Verification items for the finished model (mm, model axes). Face numbers are marked on the shaded views. A direction names the side the tool comes from. Give positions to 0.01 mm unless a question says otherwise; leave off trailing zeros. Loops run counter-clockwise (first coordinate to the right, second up) from the corner with the lowest first, then second, coordinate; pieces in that order, holes last. Notation, with made-up numbers: M 60.25,-32.5 L 79.25,-32.5 A24 ccw 79.25,-12.5 Z; hole C 13.5,12.25 d1. An arc over 180 degrees is marked long. Use a Markdown table: item, result.
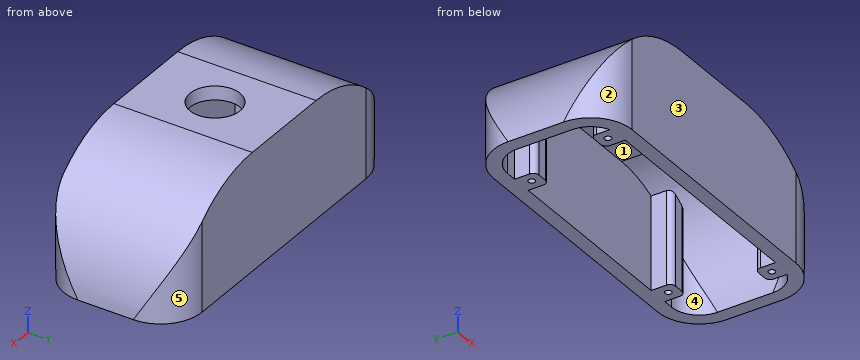
from build123d import *

# Parameters (mm, degrees)
BOSS_EXTRUDE2_DEPTH      = 44.45
BOSS_EXTRUDE2_DEPTH_BACK = 19.05
CUT_EXTRUDE_THIN1_DEPTH  = 104.419258966
SHELL1_T                 = -6.35
SKETCH5_R                = 11.5
CUT_EXTRUDE1_DEPTH       = 6.35
BOSS_EXTRUDE3_REACH      = 105.419
SKETCH8_W                = 9.525
SKETCH8_H                = 9.525
SKETCH8_R                = 1.5
FILLET1_R                = 2.54


with BuildPart() as part:
    # Sketch3 → Boss-Extrude2 (new, two sides: drawn at the far end of the back side and taken through both)
    with BuildSketch(Plane(origin=(0, 0, 0), x_dir=(1, 0, 0), z_dir=(0, 1, 0)).offset(-BOSS_EXTRUDE2_DEPTH_BACK)):
        with BuildLine():
            Line((-76.2, 0), (76.2, 0))
            ThreePointArc((76.2, 0), (60.391088515, -38.166088515), (22.225, -53.975))
            Line((22.225, -53.975), (-22.225, -53.975))
            ThreePointArc((-22.225, -53.975), (-60.391088515, -38.166088515), (-76.2, 0))
        make_face()
    extrude(amount=BOSS_EXTRUDE2_DEPTH + BOSS_EXTRUDE2_DEPTH_BACK)

    # Sketch4 → Cut-Extrude-Thin1 (cut, through all)
    with BuildSketch(Plane.XY.offset(53.975)):
        with BuildLine():
            Line((88.9, 25.4), (88.9, 0))
            ThreePointArc((88.9, 0), (79.600640303, -22.450640303), (57.15, -31.75))
            Line((57.15, -31.75), (-57.15, -31.75))
            ThreePointArc((-57.15, -31.75), (-79.600640303, -22.450640303), (-88.9, 0))
            Line((-88.9, 0), (-88.9, 25.4))
            ThreePointArc((-88.9, 25.4), (-79.600640303, 47.850640303), (-57.15, 57.15))
            Line((-57.15, 57.15), (57.15, 57.15))
            ThreePointArc((57.15, 57.15), (79.600640303, 47.850640303), (88.9, 25.4))
        make_face()
        with BuildLine():
            Line((76.2, 25.4), (76.2, 0))
            ThreePointArc((76.2, 0), (70.620384182, -13.470384182), (57.15, -19.05))
            Line((57.15, -19.05), (-57.15, -19.05))
            ThreePointArc((-57.15, -19.05), (-70.620384182, -13.470384182), (-76.2, 0))
            Line((-76.2, 0), (-76.2, 25.4))
            ThreePointArc((-76.2, 25.4), (-70.620384182, 38.870384182), (-57.15, 44.45))
            Line((-57.15, 44.45), (57.15, 44.45))
            ThreePointArc((57.15, 44.45), (70.620384182, 38.870384182), (76.2, 25.4))
        make_face(mode=Mode.SUBTRACT)
    extrude(amount=-CUT_EXTRUDE_THIN1_DEPTH, mode=Mode.SUBTRACT)

    # Shell1
    shell1_openings = [part.faces().sort_by_distance(p)[0] for p in [
        (0, 12.7, 0),
    ]]
    offset(amount=SHELL1_T, openings=shell1_openings)

    # Sketch5 → Cut-Extrude1 (cut)
    with BuildSketch(Plane.XY.offset(53.975)):
        with Locations((0, 12.7)):
            Circle(SKETCH5_R)
    extrude(amount=-CUT_EXTRUDE1_DEPTH, mode=Mode.SUBTRACT)

    # Sketch8 → Boss-Extrude3 (add, up to next)
    with BuildSketch(Plane(origin=(0, 0, 0), x_dir=(-1, 0, 0), z_dir=(0, 0, -1)), mode=Mode.PRIVATE) as boss_extrude3_sk1:
        with Locations((-47.625, 33.3375)):
            Rectangle(SKETCH8_W, SKETCH8_H)
        with Locations((-47.625, 33.3375)):
            Circle(SKETCH8_R, mode=Mode.SUBTRACT)
    boss_extrude3_tool1 = extrude(boss_extrude3_sk1.sketch, amount=-BOSS_EXTRUDE3_REACH, mode=Mode.PRIVATE) - part.part
    # Sketch8 → Boss-Extrude3 (add, up to next)
    with BuildSketch(Plane(origin=(0, 0, 0), x_dir=(-1, 0, 0), z_dir=(0, 0, -1)), mode=Mode.PRIVATE) as boss_extrude3_sk2:
        with Locations((-57.15, -7.9375)):
            Rectangle(SKETCH8_W, SKETCH8_H)
        with Locations((-57.15, -7.9375)):
            Circle(SKETCH8_R, mode=Mode.SUBTRACT)
    boss_extrude3_tool2 = extrude(boss_extrude3_sk2.sketch, amount=-BOSS_EXTRUDE3_REACH, mode=Mode.PRIVATE) - part.part
    # Sketch8 → Boss-Extrude3 (add, up to next)
    with BuildSketch(Plane(origin=(0, 0, 0), x_dir=(-1, 0, 0), z_dir=(0, 0, -1)), mode=Mode.PRIVATE) as boss_extrude3_sk3:
        with Locations((57.15, -7.9375)):
            Rectangle(SKETCH8_W, SKETCH8_H)
        with Locations((57.15, -7.9375)):
            Circle(SKETCH8_R, mode=Mode.SUBTRACT)
    boss_extrude3_tool3 = extrude(boss_extrude3_sk3.sketch, amount=-BOSS_EXTRUDE3_REACH, mode=Mode.PRIVATE) - part.part
    # Sketch8 → Boss-Extrude3 (add, up to next)
    with BuildSketch(Plane(origin=(0, 0, 0), x_dir=(-1, 0, 0), z_dir=(0, 0, -1)), mode=Mode.PRIVATE) as boss_extrude3_sk4:
        with Locations((47.625, 33.3375)):
            Rectangle(SKETCH8_W, SKETCH8_H)
        with Locations((47.625, 33.3375)):
            Circle(SKETCH8_R, mode=Mode.SUBTRACT)
    boss_extrude3_tool4 = extrude(boss_extrude3_sk4.sketch, amount=-BOSS_EXTRUDE3_REACH, mode=Mode.PRIVATE) - part.part
    add(boss_extrude3_tool1.solids().sort_by_distance((47.625, 28.709704, 0))[0])
    add(boss_extrude3_tool2.solids().sort_by_distance((57.15, -3.309704, 0))[0])
    add(boss_extrude3_tool3.solids().sort_by_distance((-52.522204, -7.9375, 0))[0])
    add(boss_extrude3_tool4.solids().sort_by_distance((-47.625, 28.709704, 0))[0])

    # Fillet1
    fillet1_edges = [part.edges().sort_by_distance(p)[0] for p in [
        (42.8625, 28.575, 21.460628012),
        (52.3875, 28.575, 18.427996491),
        (61.9125, -3.175, 13.162854637),
        (52.3875, -3.175, 18.427996491),
        (-52.3875, -3.175, 18.427996491),
        (-61.9125, -3.175, 13.162854637),
        (-52.3875, 28.575, 18.427996491),
        (-42.8625, 28.575, 21.460628012),
    ]]
    fillet(fillet1_edges, radius=FILLET1_R)


solid = part.part
(1) Cross-section at A-A on x = 0. Record the cut outline in (y, z) (3 decimals).
Results below:
| item | result |
|---|---|
| outline | M -19.05,0 L -12.7,0 L -12.7,47.625 L 1.2,47.625 L 1.2,53.975 L -19.05,53.975 Z; M 24.2,47.625 L 38.1,47.625 L 38.1,0 L 44.45,0 L 44.45,53.975 L 24.2,53.975 Z |
(2) Draft check along Y on the marked faces 3, 4 and 5. Enter one of: +Y half, -Y half, draft (parallel to the pull), parting line (faces both ways), or undercut.
Results below:
| item | result |
|---|---|
| face 3 | -Y half |
| face 4 | undercut |
| face 5 | +Y half |
(3) Set-up check for the marked faces 1 and 2: record each of +Z, -Z, +X, -X, +Y, -Y from which the full face is reachable in a straight line by a thin tool's end or side.
Results below:
| item | result |
|---|---|
| face 1 | -Z |
| face 2 | +Z, -Z, -X, -Y |
(4) Cross-section at C-C on x = 37. Record the cut outline in (y, z), then the cut area to 3 significant figures.
Results below:
| item | result |
|---|---|
| outline | M -19.05,0 L -12.7,0 L -12.7,45.28 L 38.1,45.28 L 38.1,0 L 44.45,0 L 44.45,51.91 L -19.05,51.91 Z |
| area | 997 mm^2 |
(5) Material ranges on line 1 (Y direction, x = 14, z = 24); line 2 (Y direction, x = 57, z = 23) (3 decimals); line 3 (Y direction, x = 47, z = 15.5) (3 decimals), recorded low to high.
Results below:
| item | result |
|---|---|
| line 1 | -19.05 to -12.7, 38.1 to 44.45 |
| line 2 | -19.05 to -9.43, -6.445 to -3.175, 38.1 to 44.45 |
| line 3 | -19.05 to -12.7, 28.575 to 31.974, 34.701 to 44.45 |
(6) Gauge pin test, flat ends, axial feed: P1, Ø6, axis at y = 22, z = 19.5, coming from the -X side; P2, Ø5.5, axis at y = 33, z = 15.5, coming from the -X side; P3, Ø3, axis at y = 7, z = 37.5, coming from the +X side. Record the tip position at first contact, or that the pin passes through.
Results below:
| item | result |
|---|---|
| P1 | x = -73.62 |
| P2 | x = -74.67 |
| P3 | x = 62.44 |
(7) Cross-section at B-B on y = 12.7. Record the cut outline in (x, z) (3 decimals).
Results below:
| item | result |
|---|---|
| outline | M -76.2,0 L -69.85,0 A47.625 cw -22.225,47.625 L -11.5,47.625 L -11.5,53.975 L -22.225,53.975 A53.975 ccw Z; M 11.5,47.625 L 22.225,47.625 A47.625 cw 69.85,0 L 76.2,0 A53.975 ccw 22.225,53.975 L 11.5,53.975 Z |
